```python
from build123d import *

# Parameters (mm, degrees)
RESSALTO_EXTRUS_O1_DEPTH = 10
ESBO_O1_3_R              = 1.5
RESSALTO_EXTRUS_O2_DEPTH = 2
ESBO_O2_R                = 13
CORTE_EXTRUS_O1_DEPTH    = 2
CASCA1_START             = 1.5
CASCA1_DEPTH             = 6.5
CASCA1_START_2           = 8
CASCA1_2_DEPTH           = 0.5


# Read off the part's stored shape, not the designer's step: Casca1
with BuildPart() as part:
    # Esboço1 → Ressalto-extrusão1 (new body)
    with BuildSketch(Plane.XY):
        with BuildLine():
            Line((-9, 15), (-9, 12))
            ThreePointArc((-9, 12), (-9.878679656, 9.878679656), (-12, 9))
            Line((-12, 9), (-15, 9))
            Line((-15, 9), (-15, -15))
            Line((-15, -15), (9, -15))
            Line((9, -15), (9, -12))
            ThreePointArc((9, -12), (9.878679656, -9.878679656), (12, -9))
            Line((12, -9), (15, -9))
            Line((15, -9), (15, 15))
            Line((15, 15), (-9, 15))
        make_face()
    extrude(amount=RESSALTO_EXTRUS_O1_DEPTH)

    # Esboço1<3> → Ressalto-extrusão2 (add)
    # profile 1 of 2: a face of its own
    with BuildSketch(Plane.XY):
        with BuildLine():
            ThreePointArc((-12, 9), (-9.878679656, 9.878679656), (-9, 12))
            Line((-9, 12), (-9, 15))
            Line((-9, 15), (-15, 15))
            Line((-15, 15), (-15, 9))
            Line((-15, 9), (-12, 9))
        make_face()
        with Locations((-12, 12)):
            Circle(ESBO_O1_3_R, mode=Mode.SUBTRACT)
    # profile 2 of 2: a face of its own
    with BuildSketch(Plane.XY):
        with BuildLine():
            Line((15, -15), (15, -9))
            Line((15, -9), (12, -9))
            ThreePointArc((12, -9), (9.878679656, -9.878679656), (9, -12))
            Line((9, -12), (9, -15))
            Line((9, -15), (15, -15))
        make_face()
        with Locations((12, -12)):
            Circle(ESBO_O1_3_R, mode=Mode.SUBTRACT)
    extrude(amount=RESSALTO_EXTRUS_O2_DEPTH)

    # Esboço2 → Corte-extrusão1 (cut)
    with BuildSketch(Plane.XY.offset(10)):
        Circle(ESBO_O2_R)
    extrude(amount=-CORTE_EXTRUS_O1_DEPTH, mode=Mode.SUBTRACT)

    # Casca1 outline → Casca1 (cut)
    with BuildSketch(Plane.XY.offset(CASCA1_START)):
        with BuildLine():
            Line((-13.5, -15), (7.5, -15))
            Line((7.5, -15), (7.5, -12))
            ThreePointArc((7.5, -12), (8.818019485, -8.818019485), (12, -7.5))
            Line((12, -7.5), (13.5, -7.5))
            Line((13.5, -7.5), (13.5, 13.5))
            Line((13.5, 13.5), (-7.5, 13.5))
            Line((-7.5, 13.5), (-7.5, 12))
            ThreePointArc((-7.5, 12), (-8.818019485, 8.818019485), (-12, 7.5))
            Line((-12, 7.5), (-13.5, 7.5))
            Line((-13.5, 7.5), (-13.5, -15))
        make_face()
    extrude(amount=CASCA1_DEPTH, mode=Mode.SUBTRACT)

    # Casca1 2 outline → Casca1 2 (cut)
    with BuildSketch(Plane.XY.offset(CASCA1_START_2)):
        with BuildLine():
            Line((-13.5, -5.291502622), (-13.5, -15))
            Line((-13.5, -15), (7.5, -15))
            Line((7.5, -15), (7.5, -12.409673646))
            ThreePointArc((7.5, -12.409673646), (-4.65479212, -13.732549302), (-13.5, -5.291502622))
        make_face()
        with BuildLine():
            Line((-13.5, 7.5), (-13.5, 5.291502622))
            ThreePointArc((-13.5, 5.291502622), (-13.001813807, 6.418943661), (-12.409673646, 7.5))
            Line((-12.409673646, 7.5), (-13.5, 7.5))
        make_face()
        with BuildLine():
            ThreePointArc((13.5, -5.291502622), (13.001813807, -6.418943661), (12.409673646, -7.5))
            Line((12.409673646, -7.5), (13.5, -7.5))
            Line((13.5, -7.5), (13.5, -5.291502622))
        make_face()
        with BuildLine():
            Line((-7.5, 13.5), (-7.5, 12.409673646))
            ThreePointArc((-7.5, 12.409673646), (-6.418943661, 13.001813807), (-5.291502622, 13.5))
            Line((-5.291502622, 13.5), (-7.5, 13.5))
        make_face()
        with BuildLine():
            ThreePointArc((5.291502622, 13.5), (10.253048327, 10.253048327), (13.5, 5.291502622))
            Line((13.5, 5.291502622), (13.5, 13.5))
            Line((13.5, 13.5), (5.291502622, 13.5))
        make_face()
    extrude(amount=CASCA1_2_DEPTH, mode=Mode.SUBTRACT)


solid = part.part
```
Geometry check sheet. Reference: the model listing, model coordinates, mm. A direction names the side the tool comes from. Round coordinates to 2 decimals unless told otherwise and drop trailing zeros. Order: outer loops, then holes, each group sorted by start corner. A loop starts at its lowest first (then second) coordinate and runs counter-clockwise, first axis right, second up. Notation, with made-up numbers: M -28,61.5 L -2,61.5 A8 cw -2,72.5 Z; hole C -29,31.5 d6. An arc over 180 degrees is marked long. Answer as CSV lines item,"result".
1) Sectioned sample at B-B on z = 1. Record the cut outline in (x, y), and give its area (3 significant figures).
Entries:
outline,"M -15,-15 L 15,-15 L 15,15 L -15,15 Z; hole C -12,12 d3; hole C 12,-12 d3"
area,"886 mm2"
2) Gauge pin test, flat ends, axial feed: pin 1 Ø0.9 at (y, z) = (13.5, 4.5) entering from -X; pin 2 Ø1.8 at (x, y) = (-12.5, 11) entering from +Z; pin 3 Ø1.5 at (x, y) = (-1, 5) entering from +Z. Record the tip position at first contact, or that the pin passes through.
Entries:
pin 1,"x = -9"
pin 2,"z = 2"
pin 3,"z = 1.5"
3) Tool access check on faces 1 (the face through (9.86, -9.9, 5.94)), 2 (the face through (-6.434, 12.994, 8.246)), 3 (the face through (-8.783, 8.853, 4.704)), 4 (the face through (-13, 9, 6)). Record the directions out of +Z, -Z, +X, -X, +Y, -Y that give a thin tool (end or side, any length) a straight path to the whole face; none if there is none.
Entries:
face 1,"+Z, +X, -Y"
face 2,"none"
face 3,"-Y"
face 4,"+Z, -X, +Y"
4) Sectioned sample at D-D on z = 6.5. Record the cut outline in (x, y), and give its area (3 significant figures).
Entries:
outline,"M -15,-15 L -13.5,-15 L -13.5,7.5 L -12,7.5 A4.5 ccw -7.5,12 L -7.5,13.5 L 13.5,13.5 L 13.5,-7.5 L 12,-7.5 A4.5 ccw 7.5,-12 L 7.5,-15 L 9,-15 L 9,-12 A3 cw 12,-9 L 15,-9 L 15,15 L -9,15 L -9,12 A3 cw -12,9 L -15,9 Z"
area,"135 mm2"
5) Sectioned sample at C-C on y = 0. Record the cut outline in (x, z).
Entries:
outline,"M -15,0 L 15,0 L 15,10 L 13,10 L 13,8 L 13.5,8 L 13.5,1.5 L -13.5,1.5 L -13.5,8 L -13,8 L -13,10 L -15,10 Z"
6) Mould release check, pull along Z, two halves, no side actions. Record for faces 5 (the face through (10.5, -11.93, 0.99)), 6 (the face through (-9, -10, 10)), 7 (the face through (8.783, -8.853, 4.704)): +Z half, -Z half, draft (parallel to the pull), parting line (faces both ways), or undercut.
Entries:
face 5,"draft"
face 6,"+Z half"
face 7,"undercut"
7) Sectioned sample at A-A on x = 0. Record the cut outline in (y, z).
Entries:
outline,"M -15,0 L 15,0 L 15,10 L 13,10 L 13,8 L 13.5,8 L 13.5,1.5 L -15,1.5 Z; M -15,8.5 L -14.5,8.5 L -14.5,8 L -13,8 L -13,10 L -15,10 Z"
8) Thickness scan on probe 1 along X at (y, z) = (0.5, 7.5); probe 2 along Y at (x, z) = (12, 1.1); probe 3 along X at (y, z) = (-12.25, 2.75). Record the ranges inside material, lowest first. Write a range as [from, to].
Entries:
probe 1,"[-15, -13.5], [13.5, 15]"
probe 2,"[-15, -13.5], [-10.5, 15]"
probe 3,"[-15, -13.5], [7.5, 9]"
